```python
from build123d import *

# Parameters (mm, degrees)
BOSS_EXTRUDE1_DEPTH     = 4
CUT_EXTRUDE1_DEPTH      = 49.826222463
CUT_EXTRUDE1_DEPTH_BACK = 49.826222463
SKETCH2_W               = 2
SKETCH2_H               = 4
CUT_EXTRUDE2_REACH      = 50.826
SKETCH3_R               = 1.6
FILLET1_R               = 3
CUT_EXTRUDE3_DEPTH      = 1.5


with BuildPart() as part:
    # Sketch1 → Boss-Extrude1 (new body)
    with BuildSketch(Plane(origin=(0, 0, 0), x_dir=(0, 0, -1), z_dir=(1, 0, 0))):
        with BuildLine():
            Line((0, -8), (40, -8))
            ThreePointArc((40, -8), (48, 0), (40, 8))
            Line((40, 8), (0, 8))
            ThreePointArc((0, 8), (-8, 0), (0, -8))
        make_face()
    extrude(amount=-BOSS_EXTRUDE1_DEPTH)

    # Sketch2 → Cut-Extrude1 (cut, two sides: drawn at the far end of the back side and taken through both)
    with BuildSketch(Plane.XY.offset(-CUT_EXTRUDE1_DEPTH_BACK)):
        with Locations((-1, 0)):
            Rectangle(SKETCH2_W, SKETCH2_H)
    extrude(amount=CUT_EXTRUDE1_DEPTH + CUT_EXTRUDE1_DEPTH_BACK, mode=Mode.SUBTRACT)

    # Sketch3 → Cut-Extrude2 (cut, up to next)
    with BuildSketch(Plane(origin=(0, 0, 0), x_dir=(0, 0, -1), z_dir=(1, 0, 0)), mode=Mode.PRIVATE) as cut_extrude2_sk1:
        with Locations((0, 5)):
            Circle(SKETCH3_R)
    cut_extrude2_tool1 = extrude(cut_extrude2_sk1.sketch, amount=-CUT_EXTRUDE2_REACH, mode=Mode.PRIVATE) & part.part
    # Sketch3 → Cut-Extrude2 (cut, up to next)
    with BuildSketch(Plane(origin=(0, 0, 0), x_dir=(0, 0, -1), z_dir=(1, 0, 0)), mode=Mode.PRIVATE) as cut_extrude2_sk2:
        with Locations((40, 5)):
            Circle(SKETCH3_R)
    cut_extrude2_tool2 = extrude(cut_extrude2_sk2.sketch, amount=-CUT_EXTRUDE2_REACH, mode=Mode.PRIVATE) & part.part
    # Sketch3 → Cut-Extrude2 (cut, up to next)
    with BuildSketch(Plane(origin=(0, 0, 0), x_dir=(0, 0, -1), z_dir=(1, 0, 0)), mode=Mode.PRIVATE) as cut_extrude2_sk3:
        with Locations((40, -5)):
            Circle(SKETCH3_R)
    cut_extrude2_tool3 = extrude(cut_extrude2_sk3.sketch, amount=-CUT_EXTRUDE2_REACH, mode=Mode.PRIVATE) & part.part
    # Sketch3 → Cut-Extrude2 (cut, up to next)
    with BuildSketch(Plane(origin=(0, 0, 0), x_dir=(0, 0, -1), z_dir=(1, 0, 0)), mode=Mode.PRIVATE) as cut_extrude2_sk4:
        with Locations((0, -5)):
            Circle(SKETCH3_R)
    cut_extrude2_tool4 = extrude(cut_extrude2_sk4.sketch, amount=-CUT_EXTRUDE2_REACH, mode=Mode.PRIVATE) & part.part
    # Sketch3 → Cut-Extrude2 (cut, up to next)
    with BuildSketch(Plane(origin=(0, 0, 0), x_dir=(0, 0, -1), z_dir=(1, 0, 0)), mode=Mode.PRIVATE) as cut_extrude2_sk5:
        with Locations((20, 5)):
            Circle(SKETCH3_R)
    cut_extrude2_tool5 = extrude(cut_extrude2_sk5.sketch, amount=-CUT_EXTRUDE2_REACH, mode=Mode.PRIVATE) & part.part
    # Sketch3 → Cut-Extrude2 (cut, up to next)
    with BuildSketch(Plane(origin=(0, 0, 0), x_dir=(0, 0, -1), z_dir=(1, 0, 0)), mode=Mode.PRIVATE) as cut_extrude2_sk6:
        with Locations((20, -5)):
            Circle(SKETCH3_R)
    cut_extrude2_tool6 = extrude(cut_extrude2_sk6.sketch, amount=-CUT_EXTRUDE2_REACH, mode=Mode.PRIVATE) & part.part
    add(cut_extrude2_tool1.solids().sort_by_distance((0, 5, 0))[0], mode=Mode.SUBTRACT)
    add(cut_extrude2_tool2.solids().sort_by_distance((0, 5, -40))[0], mode=Mode.SUBTRACT)
    add(cut_extrude2_tool3.solids().sort_by_distance((0, -5, -40))[0], mode=Mode.SUBTRACT)
    add(cut_extrude2_tool4.solids().sort_by_distance((0, -5, 0))[0], mode=Mode.SUBTRACT)
    add(cut_extrude2_tool5.solids().sort_by_distance((0, 5, -20))[0], mode=Mode.SUBTRACT)
    add(cut_extrude2_tool6.solids().sort_by_distance((0, -5, -20))[0], mode=Mode.SUBTRACT)

    # Fillet1
    # the kernel refuses this fillet: 3 mm, written as the material it takes off along each edge
    with BuildSketch(Plane(origin=(-4, -8, 0), x_dir=(0, 1, 0), z_dir=(0, 0, -1))) as fillet1_piece_1:
        with BuildLine():
            CenterArc((FILLET1_R, FILLET1_R), FILLET1_R, 180, 90)
            Line((0, FILLET1_R), (0, 0))
            Line((0, 0), (FILLET1_R, 0))
        make_face()
    extrude(amount=40, mode=Mode.SUBTRACT)
    with BuildSketch(Plane(origin=(-4, 0, 0), x_dir=(0, 1, 0), z_dir=(0, 0, -1))) as fillet1_piece_2:
        with BuildLine():
            CenterArc((8 - FILLET1_R, FILLET1_R), FILLET1_R, 270, 90)
            Line((8 - FILLET1_R, 0), (8, 0))
            Line((8, 0), (8, FILLET1_R))
        make_face()
    revolve(axis=Axis((-4, 0, 0), (1, 0, 0)), revolution_arc=180, mode=Mode.SUBTRACT)
    with BuildSketch(Plane(origin=(-4, 8, -40), x_dir=(1, 0, 0), z_dir=(0, 0, 1))) as fillet1_piece_3:
        with BuildLine():
            CenterArc((FILLET1_R, -FILLET1_R), FILLET1_R, 90, 90)
            Line((0, -FILLET1_R), (0, 0))
            Line((0, 0), (FILLET1_R, 0))
        make_face()
    extrude(amount=40, mode=Mode.SUBTRACT)
    with BuildSketch(Plane(origin=(-4, 0, -40), x_dir=(0, -1, 0), z_dir=(0, 0, 1))) as fillet1_piece_4:
        with BuildLine():
            CenterArc((8 - FILLET1_R, FILLET1_R), FILLET1_R, 270, 90)
            Line((8 - FILLET1_R, 0), (8, 0))
            Line((8, 0), (8, FILLET1_R))
        make_face()
    revolve(axis=Axis((-4, 0, -40), (1, 0, 0)), revolution_arc=180, mode=Mode.SUBTRACT)

    # Sketch4 → Cut-Extrude3 (cut)
    with BuildSketch(Plane.ZY.offset(4)):
        Polygon((-36.824573519, 5), (-38.41228676, 7.75), (-41.58771324, 7.75), (-43.175426481, 5), (-41.58771324, 2.25), (-38.41228676, 2.25), align=None)
        Polygon((-3.175426481, 5), (-1.58771324, 2.25), (1.58771324, 2.25), (3.175426481, 5), (1.58771324, 7.75), (-1.58771324, 7.75), align=None)
        Polygon((-3.175426481, -5), (-1.58771324, -7.75), (1.58771324, -7.75), (3.175426481, -5), (1.58771324, -2.25), (-1.58771324, -2.25), align=None)
        Polygon((-36.824573519, -5), (-38.41228676, -2.25), (-41.58771324, -2.25), (-43.175426481, -5), (-41.58771324, -7.75), (-38.41228676, -7.75), align=None)
        Polygon((-16.824573519, 5), (-18.41228676, 7.75), (-21.58771324, 7.75), (-23.175426481, 5), (-21.58771324, 2.25), (-18.41228676, 2.25), align=None)
        Polygon((-16.824573519, -5), (-18.41228676, -2.25), (-21.58771324, -2.25), (-23.175426481, -5), (-21.58771324, -7.75), (-18.41228676, -7.75), align=None)
    extrude(amount=-CUT_EXTRUDE3_DEPTH, mode=Mode.SUBTRACT)


solid = part.part
```
Design review of the part built by this model. Coordinates are the model's own, in mm. A direction names the side the tool comes from. Coordinates: 2 decimals unless noted, no trailing zeros. Order: outer loops, then holes, each group sorted by start corner. A loop starts at its lowest first (then second) coordinate and runs counter-clockwise, first axis right, second up. Notation, with made-up numbers: M 6.5,0 L 39.5,0 A19 ccw 39.5,28 Z; hole C 11.5,76 d9. An arc over 180 degrees is marked long. Answer as a JSON object with one key per item and string values. Group by question number.
1) Add section B-B, the plane y = 6. Count the separate pieces of the cut face and the enclosed holes in it, then the cut area to 3 significant figures.
2) Wall thickness on L1, parallel to Y at x = -1, z = -8; L2, parallel to Y at x = -1.15, z = -21; L3, parallel to Z at x = -0.3, y = -5.75: over which ranges is each line inside the solid? List them lowest first.
3) Add section A-A, the plane z = -20. Write out the cut boundary in (x, y), then the cut area to 3 significant figures.
4) Tool access review of faces 1 (the cylindrical face through (-1.23, -3.92, -18.82)), 2 (the flat face through (-2, 0, -20)), 3 (the flat face through (-3.1, -6, -2.6)): name each direction out of +Z, -Z, +X, -X, +Y, -Y from which nothing blocks a thin tool from reaching the whole face with its end or side.
5) Mouldability with a two-part tool opening along Y and no side actions: class faces 4 (the flat face through (0, -3, -20)), 5 (the flat face through (-0.5, 8, -20.3)), 6 (the flat face through (-3.26, 3.606, 2.37)) as pulls with the +Y half, pulls with the -Y half, needs draft (parallel to the pull), parting line crosses it, or undercut.
6) For pin 1 (0.8 mm diameter, centred on x = -3, z = -39.5, fed in from -Y); pin 2 (1.6 mm diameter, centred on x = -3, z = -20, fed in from -Y); pin 3 (0.8 mm diameter, centred on x = -3.5, z = -0.5, fed in from +Y); pin 4 (3 mm diameter, centred on y = 5, z = -20, fed in from +X), all flat-tipped, find the tip position at first contact; note any pin that passes through.
Computed values:
{
 "1": {"separate pieces": "4", "enclosed holes": "0", "area": "149 mm^2"},
 "2": {"L1": "y = -8 to -2, 2 to 8", "L2": "y = -8 to -6.25, -3.75 to -2, 2 to 3.75, 6.25 to 8", "L3": "z = -45.56 to -41.41, -38.59 to -21.41, -18.59 to -1.41, 1.41 to 5.56"},
 "3": {"outline": "M -4,-2.25 L -2.5,-2.25 L -2.5,-3.4 L 0,-3.4 L 0,-2 L -2,-2 L -2,2 L 0,2 L 0,3.4 L -2.5,3.4 L -2.5,2.25 L -4,2.25 Z; M -2.5,-7.6 A3 ccw -1,-8 L 0,-8 L 0,-6.6 L -2.5,-6.6 Z; M -2.5,6.6 L 0,6.6 L 0,8 L -1,8 A3 ccw -2.5,7.6 Z", "area": "22.4 mm^2"},
 "4": {"face 1": "+X, -X", "face 2": "+Z, -Z, +X", "face 3": "-X"},
 "5": {"face 4": "needs draft", "face 5": "pulls with the +Y half", "face 6": "undercut"},
 "6": {"pin 1": "stops at y = -2.25", "pin 2": "stops at y = -7.75", "pin 3": "stops at y = 2.25", "pin 4": "passes through"}
}
